Geometry check sheet. Reference: the model listing, model coordinates, mm. Face numbers are marked on the shaded views. Round coordinates to 2 decimals unless told otherwise and drop trailing zeros. Write each loop counter-clockwise with the first axis right and the second up, starting at its lowest first coordinate (ties: lowest second). Pieces come first, ordered by that corner, then holes. Notation, with made-up numbers: (-18, 52.25) -> (0, 52.25) arc R21 cw to (0, 74.25) -> close; hole circle Ø6 at (-30, -28). An arc over 180 degrees is marked (long way). Use a Markdown table: item, result.
Autodesk Inventor part; units mm, degrees
ref_plane "YZ Plane" through (0, 0, 0) normal (1, 0, 0) x (0, 1, 0)
ref_plane "XZ Plane" through (0, 0, 0) normal (0, 1, 0) x (-1, 0, 0)
ref_plane "XY Plane" through (0, 0, 0) normal (0, 0, 1) x (1, 0, 0)
sketch "Sketch1" plane through (0, 0, 0) normal (0, 1, 0) x (-1, 0, 0)
  line L0 (12.3825, 57.15) -> (-12.3825, 57.15)
  line L1 (-12.3825, 57.15) -> (-12.3825, -57.15)
  line L2 (-12.3825, -57.15) -> (12.3825, -57.15)
  line L3 (12.3825, -57.15) -> (12.3825, 57.15)
  line L4 (12.3825, 57.15) -> (-12.3825, -57.15) construction
  line L5 (-12.3825, 57.15) -> (12.3825, -57.15) construction
  point P0 (0, 0)
  dimension "d0" = 24.765
  dimension "d1" = 114.3
extrude "Extrusion1" add sketch "Sketch1" along normal blind 6.35
sketch "Sketch2" plane through (-12.3825, 0, 57.15) normal (0, 0, 1) x (1, 0, 0)
  line L0 (6.096, 0) -> (18.669, 0)
  line L1 (0, 0) -> (24.765, 0)
  line L2 (18.669, 0) -> (13.97, 4.699)
  line L3 (13.97, 4.699) -> (10.795, 4.699)
  line L4 (10.795, 4.699) -> (6.096, 0)
  line L5 (0, 6.35) -> (24.765, 6.35)
  point P0 (12.3825, 0)
  point P1 (12.3825, 4.699)
  point P2 (12.3825, 6.35)
  dimension "d4" = 45
  dimension "d5" = 45
  dimension "d6" = 3.175
  dimension "d7" = 4.699
extrude "Extrusion2" cut sketch "Sketch2" against normal through all
sketch "Sketch3" plane through (0, 6.35, 0) normal (0, 1, 0) x (1, 0, 0)
  line L0 (12.3825, 57.15) -> (-12.3825, 57.15) construction
  line L1 (3.175, 57.15) -> (-3.175, 57.15)
  line L2 (-3.175, 57.15) -> (-3.175, 0)
  line L3 (3.175, 0) -> (3.175, 57.15)
  arc A0 (-3.175, 0) -> (3.175, 0) centre (0, 0) ccw
  dimension "d14" = 3.175
  dimension "d15" = 57.15
extrude "Extrusion3" cut sketch "Sketch3" against normal through all
ref_plane "Work Plane1" through (12.3825, 0, -23.8125) normal (0, 0, -1) x (-1, 0, 0)
sketch "Sketch4" plane through (12.3825, 0, -23.8125) normal (0, 0, -1) x (-1, 0, 0)
  line L0 (9.2075, 3.1115) -> (9.2075, 6.35) construction
  line L1 (0, 6.35) -> (9.2075, 6.35) construction
  line L2 (0, 0) -> (0, 6.35) construction
  line L3 (0, 0) -> (6.096, 0) construction
  line L4 (6.096, 0) -> (9.2075, 3.1115) construction
  line L5 (0, 0) -> (6.096, 0)
  line L6 (1.016, 0) -> (0, 0)
  line L7 (0, 0) -> (0, 6.35)
  line L8 (0, 6.35) -> (9.2075, 6.35)
  line L9 (3.175, 6.35) -> (0, 6.35)
  line L10 (3.175, 6.35) -> (1.016, 5.1035)
  line L11 (1.016, 5.1035) -> (1.016, 0)
  point P0 (12.3825, 0)
  dimension "d19" = 150
  dimension "d20" = 1.016
  dimension "d21" = 3.175
extrude "Extrusion4" cut sketch "Sketch4" along normal mid plane 3.175
mirror "Mirror1" about plane through (0, 0, 0) normal (1, 0, 0) of "Extrusion4"
pattern_linear "Rectangular Pattern1" count 2 spacing 47.625 along (0, 0, 1) of "Extrusion4", "Mirror1"
sketch "Sketch6" plane through (-12.3825, 6.35, 57.15) normal (0, 0, 1) x (1, 0, 0)
  line L0 (6.096, -6.35) -> (10.795, -1.651) construction
  line L1 (10.795, -1.651) -> (13.97, -1.651) construction
  line L2 (13.97, -1.651) -> (18.669, -6.35) construction
  line L3 (18.669, -6.35) -> (24.765, -6.35) construction
  line L4 (24.765, -6.35) -> (24.765, 0) construction
  line L5 (0, 0) -> (24.765, 0) construction
  line L6 (0, -6.35) -> (0, 0) construction
  line L7 (0, -6.35) -> (6.096, -6.35) construction
  line L8 (9.2075, 0) -> (0, 0)
  line L9 (7.9559, 0) -> (9.4799, 1.524)
  line L10 (9.4799, 1.524) -> (15.2851, 1.524)
  line L11 (15.2851, 1.524) -> (16.8091, 0)
  line L12 (6.096, -6.35) -> (10.795, -1.651)
  line L13 (13.97, -1.651) -> (18.669, -6.35)
  line L14 (7.9559, 0) -> (16.8091, 0)
  line L15 (24.765, 0) -> (15.5575, 0)
  point P0 (12.3825, -6.35)
  point P1 (12.3825, 0)
  point P2 (12.3825, 1.524)
  dimension "d30" = 3.175
  dimension "d31" = 3.175
extrude "Extrusion5" add sketch "Sketch6" against normal blind 50.8
sketch "Sketch7" plane through (0, 6.35, 0) normal (0, 1, 0) x (1, 0, 0)
  line L0 (-9.2075, -22.225) -> (-9.2075, -25.4)
  line L1 (9.2075, -25.4) -> (9.2075, -22.225)
  line L2 (-9.2075, -25.4) -> (9.2075, -25.4)
  line L3 (9.2075, -25.4) -> (9.2075, -22.225)
  line L4 (9.2075, -22.225) -> (-9.2075, -22.225)
  line L5 (-9.2075, -22.225) -> (-9.2075, -25.4)
  point P0 (0, 0)
extrude "Extrusion6" cut sketch "Sketch7" along normal through all
sketch "Sketch8" plane through (0, 6.35, 0) normal (0, 1, 0) x (1, 0, 0)
  line L0 (12.3825, -22.225) -> (11.3665, -22.225) construction
  line L1 (11.3665, -22.225) -> (11.3665, -25.4) construction
  line L2 (11.3665, -25.4) -> (12.3825, -25.4) construction
  line L3 (12.3825, -57.15) -> (12.3825, -25.4) construction
  line L4 (6.2865, -57.15) -> (12.3825, -57.15) construction
  line L5 (6.2865, -57.15) -> (6.2865, 57.15) construction
  line L6 (12.3825, 57.15) -> (6.2865, 57.15) construction
  line L7 (12.3825, 25.4) -> (12.3825, 57.15) construction
  line L8 (12.3825, 25.4) -> (11.3665, 25.4) construction
  line L9 (11.3665, 25.4) -> (11.3665, 22.225) construction
  line L10 (11.3665, 22.225) -> (12.3825, 22.225) construction
  line L11 (12.3825, -22.225) -> (12.3825, 22.225) construction
  line L12 (-11.3665, -22.225) -> (-12.3825, -22.225) construction
  line L13 (-12.3825, 22.225) -> (-12.3825, -22.225) construction
  line L14 (-12.3825, 22.225) -> (-11.3665, 22.225) construction
  line L15 (-11.3665, 22.225) -> (-11.3665, 25.4) construction
  line L16 (-11.3665, 25.4) -> (-12.3825, 25.4) construction
  line L17 (-12.3825, 57.15) -> (-12.3825, 25.4) construction
  line L18 (-6.2865, 57.15) -> (-12.3825, 57.15) construction
  line L19 (-6.2865, 57.15) -> (-6.2865, -57.15) construction
  line L20 (-12.3825, -57.15) -> (-6.2865, -57.15) construction
  line L21 (-12.3825, -25.4) -> (-12.3825, -57.15) construction
  line L22 (-12.3825, -25.4) -> (-11.3665, -25.4) construction
  line L23 (-11.3665, -25.4) -> (-11.3665, -22.225) construction
  line L24 (-12.3825, -25.4) -> (-12.3825, -57.15)
  line L25 (-12.3825, -28.575) -> (-9.3345, -31.623)
  line L26 (-9.3345, -31.623) -> (-9.3345, -57.15)
  line L27 (-12.3825, -57.15) -> (-6.2865, -57.15)
  line L28 (-12.3825, -57.15) -> (-9.3345, -57.15)
  line L29 (-12.3825, -57.15) -> (-12.3825, -28.575)
  line L30 (-12.3825, 57.15) -> (-12.3825, 25.4) construction
  line L31 (-12.3825, 28.575) -> (-9.525, 31.4325)
  line L32 (-9.525, 31.4325) -> (-3.175, 31.4325)
  line L33 (-3.175, 57.15) -> (-3.175, 0) construction
  line L34 (-3.175, 57.15) -> (-6.2865, 57.15)
  line L35 (-3.175, 31.4325) -> (-3.175, 57.15)
  line L36 (-3.175, 57.15) -> (-12.3825, 57.15)
  line L37 (-12.3825, 28.575) -> (-12.3825, 57.15)
  point P0 (0, 0)
  dimension "d36" = 45
  dimension "d37" = 3.175
  dimension "d38" = 3.175
  dimension "d39" = 45
  dimension "d40" = 6.35
extrude "Extrusion7" cut sketch "Sketch8" against normal through all
mirror "Mirror2" about plane through (0, 0, 0) normal (1, 0, 0) of "Extrusion7"
equation "\"d38\" = d37"
equation "\"d39\" = d36"
properties part number "Holder_Slide_Top"
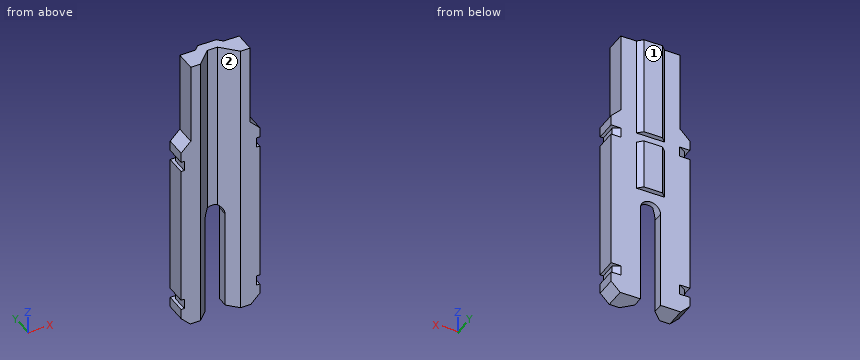
(1) Release check for a two-part mould opening along X. For the marked faces 1 and 2 record: +X half, -X half, draft (parallel to the pull), parting line (faces both ways), or undercut.
A:
| item | result |
|---|---|
| face 1 | draft |
| face 2 | undercut |
(2) Section check B-B on x = 0. Record the cut outline in (y, z) (3 decimals), plus the area to 3 significant figures.
A:
| item | result |
|---|---|
| outline | (4.699, 3.175) -> (6.35, 3.175) -> (6.35, 6.35) -> (7.874, 6.35) -> (7.874, 22.225) -> (6.35, 22.225) -> (6.35, 25.4) -> (7.874, 25.4) -> (7.874, 57.15) -> (4.699, 57.15) -> close |
| area | 162 mm2 |
(3) Gauge pin test, flat ends, axial feed: pin 1 Ø3.5 at (x, y) = (-10.5, 2) entering from +Z; pin 2 Ø1.2 at (x, y) = (1, 7) entering from -Z; pin 3 Ø1.6 at (y, z) = (3, 24) entering from +X; pin 4 Ø1.6 at (x, y) = (-10.5, 3.5) entering from +Z. Record the tip position at first contact, or that the pin passes through.
A:
| item | result |
|---|---|
| pin 1 | stops at z = 57.15 |
| pin 2 | stops at z = 6.35 |
| pin 3 | stops at x = 11.37 |
| pin 4 | stops at z = 31.26 |
(4) Section check A-A on z = 16. Record the cut outline in (x, y), plus the area to 3 significant figures.
A:
| item | result |
|---|---|
| outline | (-12.38, 0) -> (-6.29, 0) -> (-1.59, 4.7) -> (1.59, 4.7) -> (6.29, 0) -> (12.38, 0) -> (12.38, 6.35) -> (4.43, 6.35) -> (2.9, 7.87) -> (-2.9, 7.87) -> (-4.43, 6.35) -> (-12.38, 6.35) -> close |
| area | 131 mm2 |
(5) Section check D-D on x = -8. Record the cut outline in (y, z), plus the area to 4 significant figures.
A:
| item | result |
|---|---|
| outline | (0, -31.43) -> (6.35, -31.43) -> (6.35, 57.15) -> (0, 57.15) -> close |
| area | 562.5 mm2 |
(6) Section check C-C on z = 30. Record the cut outline in (x, y), plus the area to 3 significant figures.
A:
| item | result |
|---|---|
| outline | (-10.96, 0) -> (-6.29, 0) -> (-1.59, 4.7) -> (1.59, 4.7) -> (6.29, 0) -> (10.96, 0) -> (10.96, 6.35) -> (4.43, 6.35) -> (2.9, 7.87) -> (-2.9, 7.87) -> (-4.43, 6.35) -> (-10.96, 6.35) -> close |
| area | 113 mm2 |
(7) Thickness scan on line 1 (Z direction, x = -2.25, y = 7.75) (3 decimals); line 2 (Z direction, x = 10, y = 6) (1 decimal); line 3 (Y direction, x = -8.25, z = -17.5). Record the ranges inside material, lowest first.
A:
| item | result |
|---|---|
| line 1 | z = 6.35 to 22.225, 25.4 to 57.15 |
| line 2 | z = -31 to -25.4, -22.2 to 22.2, 25.4 to 31 |
| line 3 | y = 0 to 6.35 |
